Here's how the part is built. I have some questions about the finished solid (model axes, mm). Face numbers are marked on the shaded views. Round coordinates to 2 decimals unless told otherwise and drop trailing zeros. Write each loop counter-clockwise with the first axis right and the second up, starting at its lowest first coordinate (ties: lowest second). Pieces come first, ordered by that corner, then holes. Notation, with made-up numbers: (13, 5.25) - (41, 5.25) arc R18 ccw to (41, 30.25) - close; hole circle Ø5 at (73.5, -22.75). An arc over 180 degrees is marked (long way). One line per question, with ' | ' between items. Start each with the question number.
(1) Imagine slicing it at D-D (x = -22). Write out the boundary of the cut face in (y, z), plus the area to 3 significant figures.
(2) Imagine slicing it at B-B (y = 0). Give the number of separate pieces and of enclosed holes in the cut face, plus the area to 3 significant figures.
(3) If I drill on L1, parallel to Z at x = 17, y = 0; L2, parallel to Z at x = -17.75, y = 0; L3, parallel to Z at x = 7, y = 0, over which ranges is the centre line in solid material (lowest first)?
(4) Imagine slicing it at A-A (z = 0). Write out the boundary of the cut face in (x, y), plus the area to 3 significant figures.
(5) Will these pins go through, and if not, where does the flat tip stop? pin 1 (1.6 mm diameter, centred on y = 0, z = 6, fed in from -X); pin 2 (3 mm diameter, centred on x = 18.5, z = -2.5, fed in from +Y); pin 3 (4 mm diameter, centred on x = 2, z = -0.5, fed in from +Y); pin 4 (8 mm diameter, centred on x = 6.5, y = 6.5, fed in from -Z).
(6) Thinking about a two-plate mould opening in X: for the marked faces 1, 2 and 3, which applies, pulls with the +X half, pulls with the -X half, needs draft (parallel to the pull), parting line crosses it, or undercut?
(7) Imagine slicing it at C-C (x = 4). Write out the boundary of the cut face in (y, z).
Autodesk Fusion 360 part; units mm, degrees
sketch "Esquisse1" plane through (0, 0, 0) normal (0, 1, 0) x (1, 0, 0)
  line L0 (-25, -1.5) -> (-25, -15)
  line L1 (-25, -15) -> (-23, -15)
  line L2 (-23, -15) -> (-13.0387, -5)
  line L3 (-13.0387, -5) -> (12.9612, -5)
  line L4 (12.9612, -5) -> (23, -15)
  line L5 (23, -15) -> (25, -15)
  line L6 (25, -15) -> (25, -1.5)
  line L7 (25, -1.5) -> (-25, -1.5)
revolve "Révolution1" add sketch "Esquisse1" angle 360 about axis through (1.75, 0, 0) along (1, 0, 0)
sketch "Esquisse2" plane through (-25, 0, 0) normal (-1, 0, 0) x (0, -1, 0)
  circle A0 centre (0, 0) radius 15
  circle A1 centre (0, 0) radius 1.5
  line L0 (1.1208, 0.9969) -> (-1.1208, 0.9969)
  arc A2 (1.1208, 0.9969) -> (-1.1208, 0.9969) centre (0, 0) ccw
extrude "Extrusion1" add sketch "Esquisse2" against normal up to surface (50 mm away) contours A1 L0 A2
sketch "Esquisse3" plane through (-25, 0, 0) normal (-1, 0, 0) x (0, -1, 0)
  circle A0 centre (0, 0) radius 15
  arc A1 (-1.1208, 0.9969) -> (1.1208, 0.9969) centre (0, 0) ccw
  line L0 (-1.1208, 0.9969) -> (1.1208, 0.9969)
  circle A2 centre (0, 6) radius 0.9805
extrude "Extrusion2" cut sketch "Esquisse3" against normal up to surface (50 mm away) contours A2
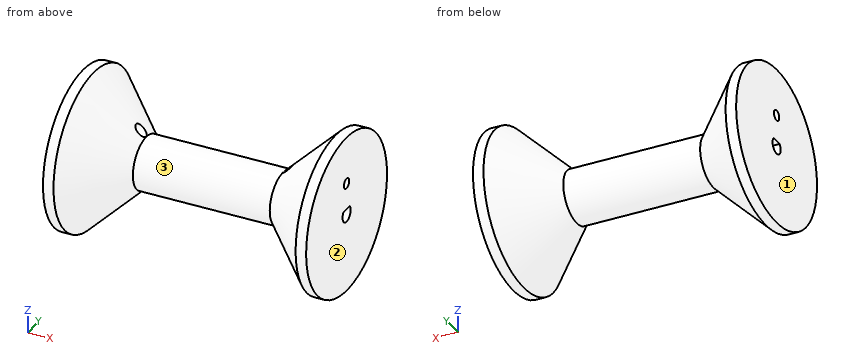
Check sheet entries:
1) outline: circle Ø27.99 at (0, 0); hole (-1.12, 1) arc R1.5 ccw (long way) to (1.12, 1) - close; hole circle Ø1.96 at (0, 6) | area: 606 mm^2
2) separate pieces: 4 | enclosed holes: 0 | area: 612 mm^2
3) L1: -9.02 to -1.5, 1 to 5.02, 6.98 to 9.02 | L2: -9.73 to -1.5, 1 to 5.02, 6.98 to 9.73 | L3: -5 to -1.5, 1 to 5
4) outline: (-25, -15) - (-23, -15) - (-13.04, -5) - (12.96, -5) - (23, -15) - (25, -15) - (25, -1.5) - (-25, -1.5) - close; (-25, 1.5) - (25, 1.5) - (25, 15) - (23, 15) - (12.96, 5) - (-13.04, 5) - (-23, 15) - (-25, 15) - close | area: 630 mm^2
5) pin 1: through | pin 2: y = 11.78 | pin 3: y = 5 | pin 4: z = -4.33
6) face 1: pulls with the -X half | face 2: pulls with the +X half | face 3: undercut
7) outline: circle Ø10 at (0, 0); hole (-1.12, 1) arc R1.5 ccw (long way) to (1.12, 1) - close
